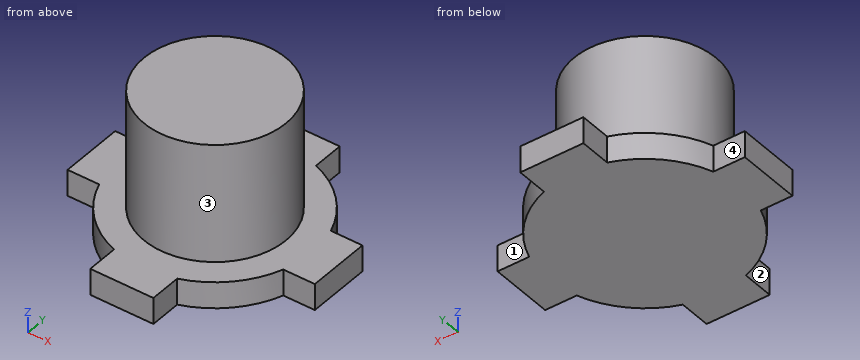
```python
from build123d import *

# Parameters (mm, degrees)
SKETCH1_R           = 2.7
BOSS_EXTRUDE1_DEPTH = 4.5
BOSS_EXTRUDE2_DEPTH = 1


with BuildPart() as part:
    # Sketch1 → Boss-Extrude1 (new body)
    with BuildSketch(Plane.XY):
        Circle(SKETCH1_R)
    extrude(amount=BOSS_EXTRUDE1_DEPTH)

    # Sketch2 → Boss-Extrude2 (add)
    with BuildSketch(Plane(origin=(0, 0, 0), x_dir=(-1, 0, 0), z_dir=(0, 0, -1))):
        with BuildLine():
            Line((-3.5, 1.2), (-4.7, 1.2))
            Line((-4.7, 1.2), (-4.7, -1.2))
            Line((-4.7, -1.2), (-3.5, -1.2))
            ThreePointArc((-3.5, -1.2), (-2.61629509, -2.61629509), (-1.2, -3.5))
            Line((-1.2, -3.5), (-1.2, -4.7))
            Line((-1.2, -4.7), (1.2, -4.7))
            Line((1.2, -4.7), (1.2, -3.5))
            ThreePointArc((1.2, -3.5), (2.61629509, -2.61629509), (3.5, -1.2))
            Line((3.5, -1.2), (4.7, -1.2))
            Line((4.7, -1.2), (4.7, 1.2))
            Line((4.7, 1.2), (3.5, 1.2))
            ThreePointArc((3.5, 1.2), (2.61629509, 2.61629509), (1.2, 3.5))
            Line((1.2, 3.5), (1.2, 4.7))
            Line((1.2, 4.7), (-1.2, 4.7))
            Line((-1.2, 4.7), (-1.2, 3.5))
            ThreePointArc((-1.2, 3.5), (-2.61629509, 2.61629509), (-3.5, 1.2))
        make_face()
    extrude(amount=BOSS_EXTRUDE2_DEPTH)


solid = part.part
```
Geometry check sheet. Reference: the model listing, model coordinates, mm. Face numbers are marked on the shaded views. A direction names the side the tool comes from. Coordinates: 2 decimals unless noted, no trailing zeros. Write each loop counter-clockwise with the first axis right and the second up, starting at its lowest first coordinate (ties: lowest second). Pieces come first, ordered by that corner, then holes. Notation, with made-up numbers: M 9,-21 L 49,-21 A28 cw 49,4 Z; hole C 19.25,-19.5 d3. An arc over 180 degrees is marked long. Use one line per item in the form item = value. Start each with the question number.
1) Set-up check for the marked faces 1, 2, 3 and 4: record each of +Z, -Z, +X, -X, +Y, -Y from which the full face is reachable in a straight line by a thin tool's end or side.
2) Section check D-D on y = -3.75. Enter the section's corners in (x, z).
3) Section check C-C on z = 1.3. Enter the section's corners in (x, y), and give its area (3 significant figures).
4) Go/stop test with flat-tipped pins: pin 1 Ø0.8 at (x, z) = (4, -0.5) entering from +Y; pin 2 Ø5 at (x, y) = (2, -2.5) entering from +Z; pin 3 Ø3 at (y, z) = (3.5, -0.5) entering from +X; pin 4 Ø0.5 at (y, z) = (-4, -0.5) entering from -X. Record where each tip stops, or that it passes through.
5) Section check A-A on y = 0. Enter the section's corners in (x, z), and give its area (3 significant figures).
6) Thickness scan on probe 1 along Z at (x, y) = (3, 0); probe 2 along Y at (x, z) = (-2, 3.25); probe 3 along Y at (x, z) = (0.25, 3.15). Record the ranges inside material, lowest first. Write a range as from..to.
Responses:
q1.face_1 = +Z, -Z, +X, +Y
q1.face_2 = +Z, -Z, -X, -Y
q1.face_3 = +Z
q1.face_4 = +Z, -Z, -X, +Y
q2.outline = M -1.2,-1 L 1.2,-1 L 1.2,0 L -1.2,0 Z
q3.outline = C 0,0 d5.4
q3.area = 22.9 mm2
q4.pin_1 = 1.2
q4.pin_2 = 4.5
q4.pin_3 = 3.11
q4.pin_4 = -1.2
q5.outline = M -4.7,-1 L 4.7,-1 L 4.7,0 L 2.7,0 L 2.7,4.5 L -2.7,4.5 L -2.7,0 L -4.7,0 Z
q5.area = 33.7 mm2
q6.probe_1 = -1..0
q6.probe_2 = -1.81..1.81
q6.probe_3 = -2.69..2.69
